from build123d import *

# Parameters (mm, degrees)
SKETCH_W        = 406
SKETCH_H        = 252
PAD_DEPTH       = 20
SKETCH001_W     = 385
SKETCH001_H     = 233
POCKET_DEPTH    = 15
SKETCH002_R     = 4
SKETCH002_R_2   = 5
SKETCH002_R_3   = 5.5
POCKET001_DEPTH = 5.001


with BuildPart() as part:
    # Sketch → Pad (new body)
    with BuildSketch(Plane.XY):
        with Locations((203, 126)):
            Rectangle(SKETCH_W, SKETCH_H)
    extrude(amount=PAD_DEPTH)

    # Sketch001 (on Face5 of Pad) → Pocket (cut)
    with BuildSketch(Plane(origin=(0, 0, 0), x_dir=(1, 0, 0), z_dir=(0, 0, -1))):
        with Locations((195.5, -124.5)):
            Rectangle(SKETCH001_W, SKETCH001_H)
    extrude(amount=-POCKET_DEPTH, mode=Mode.SUBTRACT)

    # Sketch002 (on Face11 of Pocket) → Pocket001 (cut, through all)
    with BuildSketch(Plane(origin=(0, 0, 15), x_dir=(1, 0, 0), z_dir=(0, 0, -1))):
        with Locations((23, -201)):
            Circle(SKETCH002_R)
        with Locations((23, -124.5)):
            Circle(SKETCH002_R_2)
        with Locations((23, -48)):
            Circle(SKETCH002_R)
        with Locations((366, -124.5)):
            Circle(SKETCH002_R_3)
    extrude(amount=-POCKET001_DEPTH, mode=Mode.SUBTRACT)


solid = part.part
Verification items for the finished model (mm, model axes). A direction names the side the tool comes from. Coordinates: 2 decimals unless noted, no trailing zeros. Order: outer loops, then holes, each group sorted by start corner. A loop starts at its lowest first (then second) coordinate and runs counter-clockwise, first axis right, second up. Notation, with made-up numbers: M -7,69 L 4,69 A33 cw 4,99 Z; hole C 82.5,50 d11. An arc over 180 degrees is marked long. One line per item, written item: value. Start each with the question number.
Item 1: Sectioned sample at A-A (y = 124.5). Enter the section's corners in (x, z), then the cut area to 3 significant figures.
Item 2: Sectioned sample at D-D (x = 23). Enter the section's corners in (y, z).
Item 3: Gauge pin test, flat ends, axial feed: pin 1 (10.5 mm diameter, centred on x = 23, y = 201, fed in from -Z); pin 2 (5 mm diameter, centred on x = 319.5, z = 2.5, fed in from -Y). Record the tip position at first contact, or that the pin passes through.
Item 4: Sectioned sample at C-C (x = 366). Enter the section's corners in (y, z).
Item 5: Mould release check, pull along X, two halves, no side actions. Record for faces 3 (the flat face through (0, 124, 10)), 4 (the flat face through (406, 124, 10)), 5 (the cylindrical face through (371.246, 122.848, 17.465)), 6 (the flat face through (262, 5, 0)): released by +X, released by -X, zero draft, split by the parting line, or undercut.
Item 6: Sectioned sample at B-B (z = 7.5). Enter the section's corners in (x, y), then the cut area to 3 significant figures.
Item 7: Scan lines: probe 1 along Y at (x, z) = (23, 18.3); probe 2 along X at (y, z) = (124.5, 18.65); probe 3 along X at (y, z) = (48, 18.65). Record each from-to range of solid material in increasing order.
Item 8: Access from +Z, -Z, +X, -X, +Y, -Y to the whole of each face (thin tool, end or side, straight path). Record for faces 1 (the flat face through (200, 0, 10)), 2 (the flat face through (193, 241, 7)).
Conclusion:
1. outline: M 0,0 L 3,0 L 3,15 L 18,15 L 18,20 L 0,20 Z; M 28,15 L 360.5,15 L 360.5,20 L 28,20 Z; M 371.5,15 L 388,15 L 388,0 L 406,0 L 406,20 L 371.5,20 Z
1. area: 2,240 mm^2
2. outline: M 0,0 L 8,0 L 8,15 L 44,15 L 44,20 L 0,20 Z; M 52,15 L 119.5,15 L 119.5,20 L 52,20 Z; M 129.5,15 L 197,15 L 197,20 L 129.5,20 Z; M 205,15 L 241,15 L 241,0 L 252,0 L 252,20 L 205,20 Z
3. pin 1: stops at z = 15
3. pin 2: stops at y = 0
4. outline: M 0,0 L 8,0 L 8,15 L 119,15 L 119,20 L 0,20 Z; M 130,15 L 241,15 L 241,0 L 252,0 L 252,20 L 130,20 Z
5. face 3: released by -X
5. face 4: released by +X
5. face 5: undercut
5. face 6: zero draft
6. outline: M 0,0 L 406,0 L 406,252 L 0,252 Z; hole M 3,8 L 388,8 L 388,241 L 3,241 Z
6. area: 12,600 mm^2
7. probe 1: y = 0 to 44, 52 to 119.5, 129.5 to 197, 205 to 252
7. probe 2: x = 0 to 18, 28 to 360.5, 371.5 to 406
7. probe 3: x = 0 to 19, 27 to 406
8. face 1: +Z, -Z, +X, -X, -Y
8. face 2: -Z
